Check sheet for the modelled part. Datum: model origin and axes. Units: mm. A direction names the side the tool comes from. Give positions to 0.01 mm unless a question says otherwise; leave off trailing zeros. Order: outer loops, then holes, each group sorted by start corner. A loop starts at its lowest first (then second) coordinate and runs counter-clockwise, first axis right, second up.
Autodesk Inventor part; units mm, degrees
ref_plane "YZ Plane" through (0, 0, 0) normal (1, 0, 0) x (0, 1, 0)
ref_plane "XZ Plane" through (0, 0, 0) normal (0, 1, 0) x (-1, 0, 0)
ref_plane "XY Plane" through (0, 0, 0) normal (0, 0, 1) x (1, 0, 0)
sketch "Sketch1" plane through (0, 0, 0) normal (0, 0, 1) x (1, 0, 0)
  line L0 (0, 0) -> (25, 0)
  line L1 (25, 0) -> (25, 40)
  line L2 (25, 40) -> (0, 40)
  line L3 (0, 40) -> (0, 0)
  dimension "d1" = 25
  dimension "d2" = 40
  dimension "d3" = 25
extrude "Extrusion1" add sketch "Sketch1" against normal blind 30
sketch "Sketch2" plane through (25, 0, 0) normal (1, 0, 0) x (0, 0, -1)
  line L0 (0, 0) -> (30, 0)
  circle A0 centre (15, 6.56) radius 2.46
extrude "Extrusion2" cut sketch "Sketch2" against normal blind 30
sketch "Sketch3" plane through (0, 0, 0) normal (-1, 0, 0) x (0, 0, 1)
  line L0 (0, 0) -> (-30, 0)
  line L1 (-25.05, 0) -> (-4.95, 0)
  line L2 (-4.95, 0) -> (-4.95, 33.12)
  line L3 (-4.95, 33.12) -> (-25.05, 33.12)
  line L4 (-25.05, 33.12) -> (-25.05, 0)
  dimension "d11" = 20.1
extrude "Extrusion3" cut sketch "Sketch3" against normal blind 20
sketch "Sketch4" plane through (0, 0, 0) normal (0, -1, 0) x (1, 0, 0)
  line L0 (20, -4.95) -> (20, -25.05)
  line L1 (20, -15) -> (25, -15)
  line L2 (25, 0) -> (25, -30)
  line L3 (20, -8.025) -> (25, -8.025)
  line L4 (25, -8.025) -> (25, -21.975)
  line L5 (25, -21.975) -> (20, -21.975)
  line L6 (20, -21.975) -> (20, -8.025)
  line L7 (20, -8.025) -> (25, -21.975) construction
  line L8 (25, -8.025) -> (20, -21.975) construction
  line L9 (25, -12.54) -> (25, -17.46)
  point P0 (0, 0)
  point P1 (22.5, -15)
  dimension "d14" = 13.95
extrude "Extrusion4" add sketch "Sketch4" along normal blind 15
sketch "Sketch5" plane through (20, 0, 0) normal (-1, 0, 0) x (0, 0, 1)
  circle A0 centre (-15, 6.56) radius 2.46
  circle A1 centre (-15, 6.56) radius 4.7025
  circle A2 centre (-15, 6.56) radius 2.46
  circle A3 centre (-15, 6.56) radius 2.46
  point P0 (0, 0)
  dimension "d17" = 9.405
extrude "Extrusion5" cut sketch "Sketch5" against normal blind 2.1
sketch "Sketch6" plane through (25, 0, 0) normal (1, 0, 0) x (0, 0, -1)
  circle A0 centre (15, 6.56) radius 4.7025
  line L0 (15, 6.56) -> (15, 23.56)
  circle A1 centre (15, 23.56) radius 2.46
  point P0 (0, 0)
  dimension "d20" = 17
  dimension "d21" = 4.92
extrude "Extrusion6" cut sketch "Sketch6" against normal blind 10 contours A1
sketch "Sketch7" plane through (20, 0, 0) normal (-1, 0, 0) x (0, 0, 1)
  circle A0 centre (-15, 23.56) radius 2.46
  circle A1 centre (-15, 23.56) radius 4.7025
  point P0 (0, 0)
  dimension "d24" = 9.405
extrude "Extrusion7" cut sketch "Sketch7" against normal blind 2.1
sketch "Sketch9" plane through (25, 0, 0) normal (1, 0, 0) x (0, 0, -1)
  circle A0 centre (15, 6.56) radius 2.46
  circle A1 centre (15, 6.56) radius 2.46
  circle A2 centre (15, 23.56) radius 2.46
  circle A3 centre (15, 23.56) radius 2.46
  line L0 (30, 40) -> (30, 0)
  line L1 (30, 0) -> (30, 40)
  line L2 (30, 40) -> (0, 40)
  line L3 (0, 40) -> (0, 0)
  line L4 (0, 0) -> (8.025, 0)
  line L5 (21.975, 0) -> (21.975, -15)
  line L6 (21.975, -15) -> (8.025, -15)
  line L7 (8.025, -15) -> (8.025, 0)
  line L8 (0, 0) -> (8.025, 0)
  line L9 (21.975, 0) -> (30, 0)
extrude "Extrusion8" add sketch "Sketch9" along normal blind 5
sketch "Sketch10" plane through (0, 40, 0) normal (0, 1, 0) x (1, 0, 0)
  line L0 (0, 30) -> (30, 30)
  line L1 (30, 0) -> (0, 0)
  line L2 (0, 30) -> (30, 30)
  line L3 (30, 30) -> (30, 0)
  line L4 (30, 0) -> (0, 0)
  line L5 (0, 0) -> (0, 30)
extrude "Extrusion9" add sketch "Sketch10" along normal blind 30
sketch "Sketch12" plane through (30, 0, 0) normal (1, 0, 0) x (0, 0, -1)
  circle A0 centre (15, 6.56) radius 2.46
  line L0 (15, 6.56) -> (15, 15.06)
  circle A1 centre (15, 15.06) radius 2.525
  point P0 (0, 0)
  dimension "d31" = 8.5
  dimension "d33" = 5.05
extrude "Extrusion10" cut sketch "Sketch12" against normal blind 30 contours A1
sketch "Sketch15" plane through (0, 0, -25.05) normal (-1, 0, 0) x (0, 0, 1)
  line L0 (0, 33.12) -> (20.1, 33.12)
  line L1 (20.1, 33.12) -> (20.1, 0)
  line L2 (0, 33.12) -> (20.1, 33.12)
  line L3 (20.1, 33.12) -> (20.1, 31.1)
  line L4 (20.1, 31.1) -> (0, 31.1)
  line L5 (0, 31.1) -> (0, 33.12)
  point P0 (25.05, 0)
  dimension "d57" = 2.02
extrude "Extrusion13" add sketch "Sketch15" against normal blind 20
sketch "Sketch17" plane through (0, 0, 0) normal (0, 0, 1) x (1, 0, 0)
  line L0 (0, 70) -> (30, 70)
  line L1 (30, 70) -> (50.0622, 90.0622)
  line L2 (30, 70) -> (80, 70) construction
  line L3 (11.9522, 97.2454) -> (0, 85.2932)
  line L4 (0, 70) -> (0, 85.2932)
  line L5 (0, 70) -> (0, 0)
  line L6 (0, 70) -> (30, 70)
  line L7 (10.923, 112.2849) -> (0, 120.567)
  line L8 (50.0622, 105.3553) -> (50.0622, 120.567)
  line L9 (50.0622, 105.3553) -> (50.0622, 90.0622)
  arc A0 (11.9522, 97.2454) -> (10.923, 112.2849) centre (4.8811, 104.3165) ccw
  line L10 (0, 150.567) -> (30, 150.567)
  line L11 (30, 150.567) -> (50.0622, 120.567)
  line L12 (5, 147.567) -> (0, 150.567)
  line L13 (5, 123.567) -> (0, 120.567)
  line L14 (5, 123.567) -> (10, 135.567)
  line L15 (10, 135.567) -> (5, 147.567)
  dimension "d61" = 45
  dimension "d62" = 32.0271
  dimension "d72" = 10
extrude "Extrusion14" add sketch "Sketch17" against normal blind 30
properties part number "rec_c_24mm_x_30mm"
1) Section check A-A, the plane y = 15.06. Record the cut outline in (x, z) (3 decimals), then the cut area to 4 significant figures.
Recorded:
outline: (0, -30) - (30, -30) - (30, -17.525) - (20, -17.525) - (20, -25.05) - (0, -25.05) - close; (0, -4.95) - (20, -4.95) - (20, -12.475) - (30, -12.475) - (30, 0) - (0, 0) - close
area: 447.5 mm2
2) Section check B-B, the plane y = -2. Record the cut outline in (x, z) (3 decimals), then the cut area to 4 significant figures.
Recorded:
outline: (20, -21.975) - (30, -21.975) - (30, -8.025) - (20, -8.025) - close
area: 139.5 mm2
3) Material ranges on L1, parallel to Y at x = 26.5, z = -15 (3 decimals); L2, parallel to Z at x = 28, y = 23.56; L3, parallel to Y at x = 5, z = -24.25, recorded low to high.
Recorded:
L1: y = -15 to 4.1, 9.02 to 12.535, 17.585 to 21.1, 26.02 to 150.567
L2: z = -30 to -17.46, -12.54 to 0
L3: y = 31.1 to 90.29, 116.78 to 123.57, 147.57 to 150.57
4) Draft check along Y on faces 1 (the face through (39.89, 135.78, -14.79)), 2 (the face through (2.535, 122.088, -14.79)), 3 (the face through (10, 31.1, -15)). Enter one of: +Y half, -Y half, draft (parallel to the pull), parting line (faces both ways), or undercut.
Recorded:
face 1: +Y half
face 2: undercut
face 3: -Y half
5) Section check C-C, the plane x = 35. Record the cut outline in (y, z).
Recorded:
outline: (75, -30) - (143.09, -30) - (143.09, 0) - (75, 0) - close
6) Depth check by flat-ended pin: pin 1 Ø3 at (x, y) = (24.5, -8.5) entering from +Z (3 decimals); pin 2 Ø7.5 at (y, z) = (5.5, -17) entering from -X; pin 3 Ø4 at (x, z) = (22, -27) entering from -Y; pin 4 Ø3 at (y, z) = (23.56, -15) entering from -X. Enter the tip coordinate at first touch or a pass-through.
Recorded:
pin 1: stops at z = -8.025
pin 2: stops at x = 20
pin 3: stops at y = 0
pin 4: passes through
7) Set-up check for faces 4 (the face through (22.1, 21.5, -13)), 5 (the face through (25, -7, -21.975)), 6 (the face through (7.465, 129.483, -14.79)), 7 (the face through (25, -8, -8.025)): record each of +Z, -Z, +X, -X, +Y, -Y from which the full face is reachable in a straight line by a thin tool's end or side.
Recorded:
face 4: -X
face 5: -Z, +X, -X, -Y
face 6: +Z, -Z, -X
face 7: +Z, +X, -X, -Y
